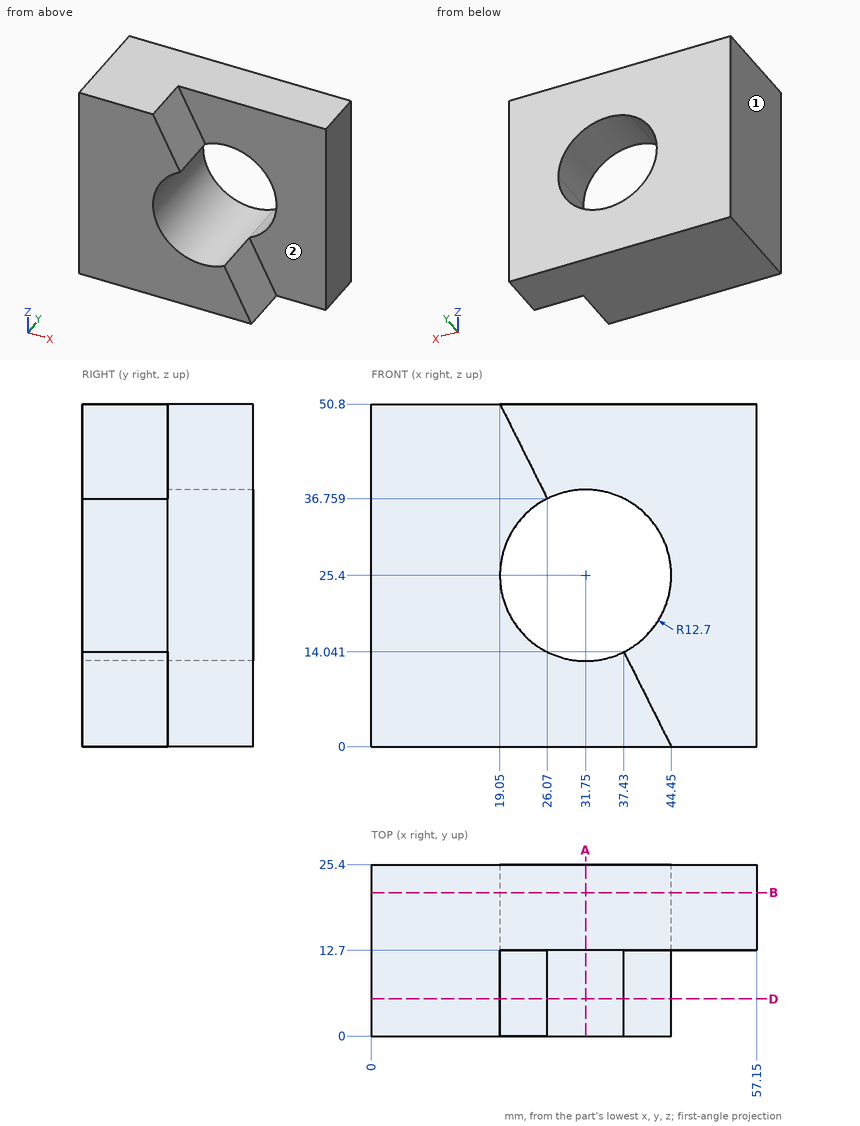
Check sheet for the drawn part. Datum: minimum x, y, z corner. Units: mm. A direction names the side the tool comes from. Give positions to 0.01 mm unless a question says otherwise; leave off trailing zeros. Loops run counter-clockwise (first coordinate to the right, second up) from the corner with the lowest first, then second, coordinate; pieces in that order, holes last.
1) Depth check by flat-ended pin: pin 1 Ø6 at (x, z) = (28, 17.5) entering from +Y; pin 2 Ø3 at (y, z) = (7.5, 29.5) entering from +X; pin 3 Ø11.5 at (x, z) = (38.5, 29) entering from -Y. Enter the tip coordinate at first touch or a pass-through.
2) Sectioned sample at D-D, the plane y = 5.5. Enter the section's corners in (x, z), then the cut area to 3 significant figures.
3) Sectioned sample at A-A, the plane x = 31.75. Enter the section's corners in (y, z), then the cut area to 3 significant figures.
4) Thickness scan on line 1 along Y through (x, z) = (43.5, 40.5); line 2 along Z through (x, y) = (24.5, 23.25); line 3 along X through (y, z) = (16.5, 31.5). Record the ranges inside material, lowest first.
5) Set-up check for the marked faces 1 and 2: record each of +Z, -Z, +X, -X, +Y, -Y from which the full face is reachable in a straight line by a thin tool's end or side.
6) Sectioned sample at B-B, the plane y = 21.25. Enter the section's corners in (x, z).
Answers:
1. pin 1: passes through
1. pin 2: stops at x = 20.35
1. pin 3: stops at y = 12.7
2. outline: (0, 0) - (44.45, 0) - (37.43, 14.04) arc R12.7 cw to (26.07, 36.76) - (19.05, 50.8) - (0, 50.8) - close
2. area: 1,360 mm2
3. outline: (0, 0) - (25.4, 0) - (25.4, 12.7) - (0, 12.7) - close; (12.7, 38.1) - (25.4, 38.1) - (25.4, 50.8) - (12.7, 50.8) - close
3. area: 484 mm2
4. line 1: y = 12.7 to 25.4
4. line 2: z = 0 to 14.97, 35.83 to 50.8
4. line 3: x = 0 to 20.61, 42.89 to 57.15
5. face 1: +Z, -Z, -X, +Y, -Y
5. face 2: +Z, +X, -Y
6. outline: (0, 0) - (57.15, 0) - (57.15, 50.8) - (0, 50.8) - close; hole circle Ø25.4 at (31.75, 25.4)
